The listing builds one solid part. Answer for the finished solid, in the listing's coordinates (mm). Round coordinates to 2 decimals unless told otherwise and drop trailing zeros. Write each loop counter-clockwise with the first axis right and the second up, starting at its lowest first coordinate (ties: lowest second). Pieces come first, ordered by that corner, then holes. Notation, with made-up numbers: (54, 0) - (77, 0) arc R33 cw to (77, 39) - close; hole circle Ø8 at (49, -10). An arc over 180 degrees is marked (long way). Answer in a Markdown table with one row per item.
Autodesk Inventor part; units mm, degrees
ref_plane "YZ Plane" through (0, 0, 0) normal (1, 0, 0) x (0, 1, 0)
ref_plane "XZ Plane" through (0, 0, 0) normal (0, 1, 0) x (-1, 0, 0)
ref_plane "XY Plane" through (0, 0, 0) normal (0, 0, 1) x (1, 0, 0)
sketch "Sketch1" plane through (0, 0, 0) normal (0, 0, 1) x (1, 0, 0)
  line L0 (0, 0) -> (23.76, 0)
  line L1 (23.76, 0) -> (23.76, 27)
  line L2 (23.76, 27) -> (0, 27)
  line L3 (0, 27) -> (0, 0)
  dimension "d0" = 23.76
  dimension "d1" = 27
extrude "Extrusion1" add sketch "Sketch1" along normal blind 1
sketch "Sketch3" plane through (23.76, 0, 0) normal (1, 0, 0) x (0, 0, -1)
  line L0 (-1, 0) -> (-1, 27)
  line L1 (0, 0) -> (-1, 0)
  line L2 (0, 0) -> (0, 27)
  line L3 (0, 27) -> (-1, 27)
  circle A0 centre (-0.8098, 23.2257) radius 0.4098
  line L4 (-0.4, 23.7) -> (-0.4, 16.95)
  point P0 (0, 0)
extrude "Extrusion3" cut sketch "Sketch3" against normal through all contours A0 L0 | L0 A0
pattern_linear "Rectangular Pattern2" count 10 spacing 1 along (0, -1, 0) of "Extrusion3"
properties part number "00_chip_fibers_01"
(1) Section A-A (x = 8.25) is taken. Give the vertices of the cut face in (y, z).
Checked values:
| item | result |
|---|---|
| outline | (0, 0) - (27, 0) - (27, 1) - (23.59, 1) arc R0.41 cw (long way) to (22.86, 1) - (22.59, 1) arc R0.41 cw (long way) to (21.86, 1) - (21.59, 1) arc R0.41 cw (long way) to (20.86, 1) - (20.59, 1) arc R0.41 cw (long way) to (19.86, 1) - (19.59, 1) arc R0.41 cw (long way) to (18.86, 1) - (18.59, 1) arc R0.41 cw (long way) to (17.86, 1) - (17.59, 1) arc R0.41 cw (long way) to (16.86, 1) - (16.59, 1) arc R0.41 cw (long way) to (15.86, 1) - (15.59, 1) arc R0.41 cw (long way) to (14.86, 1) - (14.59, 1) arc R0.41 cw (long way) to (13.86, 1) - (0, 1) - close |
(2) A flat-ended cylindrical pin translates along its axis: pin 1 (3 mm diameter, centred on x = 10.5, y = 15, fed in from +Z). Find the tip coordinate at first contact, or state that the pin passes through.
Checked values:
| item | result |
|---|---|
| pin 1 | stops at z = 1 |
(3) Find the intervals of material crossed by line 1 (Z direction, x = 10.75, y = 23.5), in increasing order.
Checked values:
| item | result |
|---|---|
| line 1 | z = 0 to 0.51 |
(4) For a pull along Y with two mould halves and no side action, classify faces 1 (the flat face through (12, 25, 1)), 2 (the cylindrical face through (12, 23.2, 0.4)), 3 (the flat face through (11.7, 0, 0.5)) as pulls with the +Y half, pulls with the -Y half, needs draft (parallel to the pull), parting line crosses it, or undercut.
Checked values:
| item | result |
|---|---|
| face 1 | needs draft |
| face 2 | undercut |
| face 3 | pulls with the -Y half |
(5) Section B-B (z = 0.85) is taken. State how many separate pieces and enclosed holes the cut face has, and give its area (3 significant figures).
Checked values:
| item | result |
|---|---|
| separate pieces | 11 |
| enclosed holes | 0 |
| area | 448 mm2 |
